Geometry: final body of the model. Coordinates: model frame, mm. A direction names the side the tool comes from. Round coordinates to 2 decimals unless told otherwise and drop trailing zeros. Loops run counter-clockwise (first coordinate to the right, second up) from the corner with the lowest first, then second, coordinate; pieces in that order, holes last. Notation, with made-up numbers: (74.5, 50) - (111.5, 50) arc R20 cw to (111.5, 74) - close; hole circle Ø1 at (68.5, -38). An arc over 180 degrees is marked (long way). Answer as CSV lines item,"result".
Autodesk Inventor part; units mm, degrees
ref_plane "Work Plane1" through (0, 0, 0) normal (0, 0, 1) x (1, 0, 0)
ref_plane "Work Plane2" through (0, 0, 0) normal (0, 0, 1) x (1, 0, 0)
ref_plane "YZ Plane" through (0, 0, 0) normal (1, 0, 0) x (0, 1, 0)
ref_plane "Work Plane1" through (0, 0, 0) normal (0, 0, 1) x (1, 0, 0)
sketch "Sketch1" plane through (0, 0, 0) normal (0, 0, 1) x (1, 0, 0)
  line L0 (-0.2674, 6.35) -> (2.5266, 6.35)
  line L1 (2.5266, 6.35) -> (2.5266, -6.35)
  line L2 (2.9076, -6.35) -> (-0.2674, -6.35)
  line L3 (-0.2674, -6.35) -> (-0.2674, 6.35)
  line L4 (2.5266, -6.35) -> (-0.2674, -6.35)
  line L5 (-0.2674, -6.35) -> (-0.2674, 6.35)
  line L6 (-0.2674, 6.35) -> (2.5266, 6.35)
  line L7 (2.5266, 6.35) -> (2.5266, -6.35)
  point P0 (0, 0)
  dimension "d0" = 2.794
  dimension "d1" = 12.7
extrude "Extrusion1" add sketch "Sketch1" against normal blind 12.7
ref_plane "Work Plane2" through (0, 0, 0) normal (0, 0, 1) x (1, 0, 0)
sketch "Sketch2" plane through (0, 0, 0) normal (0, 0, 1) x (1, 0, 0)
  line L0 (2.9076, -6.35) -> (-0.2674, -6.35)
  line L1 (-0.2674, -6.35) -> (-0.2674, 6.35)
  line L2 (-0.2674, 6.35) -> (2.9076, 6.35)
  line L3 (2.9076, 10.3713) -> (2.9076, 6.35)
  line L4 (2.9076, -6.35) -> (2.9076, -10.3713)
  line L5 (-0.2674, 6.35) -> (-0.2674, -6.35)
  line L6 (-0.2674, -6.35) -> (2.5266, -6.35)
  line L7 (2.5266, -6.35) -> (2.5266, 6.35)
  line L8 (2.5266, 6.35) -> (-0.2674, 6.35)
  line L9 (-0.2674, 6.35) -> (2.9076, 6.35)
  line L10 (2.9076, 6.35) -> (2.9076, -6.35)
  line L11 (2.9076, -6.35) -> (-0.2674, -6.35)
  line L12 (-0.2674, -6.35) -> (-0.2674, 6.35)
  line L13 (6.0826, -12.065) -> (-0.0044, -12.065)
  line L14 (-0.0044, 12.065) -> (6.0826, 12.065)
  line L15 (-2.8074, 9.262) -> (-0.0044, 12.065)
  line L16 (-2.8074, -9.262) -> (-2.8074, 9.262)
  line L17 (-0.0044, -12.065) -> (-2.8074, -9.262)
  line L18 (6.0826, -12.065) -> (6.0826, -10.3713) construction
  line L19 (2.9076, -10.3713) -> (6.0826, -10.3713)
  line L20 (6.0826, 10.3713) -> (2.9076, 10.3713)
  line L21 (6.0826, 10.3713) -> (6.0826, 12.065) construction
  line L22 (2.9076, -10.3713) -> (2.9076, -12.065)
  line L23 (2.9076, 10.3713) -> (2.9076, 12.065)
  point P0 (0, 0)
extrude "Extrusion2" add sketch "Sketch2" along normal blind 3.175
chamfer "Chamfer1" distance 0.635 angle 45 15 edges at (-1.4059, 10.6635, 3.175) (1.4516, 12.065, 3.175) (-2.8074, 0, 3.175) (-1.4059, -10.6635, 3.175) (1.4516, -12.065, 3.175) (1.4516, 12.065, 0) (1.4516, -12.065, 0) (-1.4059, -10.6635, 0) (-2.8074, 0, 0) (-1.4059, 10.6635, 0) (2.9076, 12.065, 1.5875) (2.9076, -12.065, 1.5875) (2.9076, 0, 3.175) (1.1296, 6.35, -12.7) (1.1296, -6.35, -12.7)
properties part number "3114a_Coil Sleeve Lock_V1" material "Acetal Resin, White"
(1) Material intervals for line 1 along X through (y, z) = (4.5, -10.25); line 2 along Y through (x, z) = (-0.1, -9.5); line 3 along Z through (x, y) = (-1.5, 1.75) (3 decimals), sorted ascending.
Findings below:
line 1,"-0.27 to 2.53"
line 2,"-6.35 to 6.35"
line 3,"0 to 3.175"
(2) Section B-B (x = 1.8). Output: boundary loops of the cut face in (y, z) (3 decimals).
Findings below:
outline,"(-12.065, 0.635) - (-11.43, 0) - (-6.35, 0) - (-6.35, -12.065) - (-5.715, -12.7) - (5.715, -12.7) - (6.35, -12.065) - (6.35, 0) - (11.43, 0) - (12.065, 0.635) - (12.065, 2.54) - (11.43, 3.175) - (-11.43, 3.175) - (-12.065, 2.54) - close"
(3) Pin query (flat end, axial travel): P1, Ø2, axis at x = 1, z = -6, coming from the -Y side; P2, Ø5, axis at y = 0.5, z = -11, coming from the +X side; P3, Ø3, axis at x = 0.5, z = -8.5, coming from the +Y side. Return the tip coordinate at first contact, or that it passes through.
Findings below:
P1,"y = -6.35"
P2,"x = 2.53"
P3,"y = 6.35"
(4) Section A-A (y = 1.5). Output: boundary loops of the cut face in (x, z) (3 decimals).
Findings below:
outline,"(-2.807, 0.635) - (-2.172, 0) - (-0.267, 0) - (-0.267, -12.7) - (2.527, -12.7) - (2.527, 0) - (2.908, 0) - (2.908, 2.54) - (2.273, 3.175) - (-2.172, 3.175) - (-2.807, 2.54) - close"
(5) Access query for faces 1 (the face through (1, 6.35, -6)), 2 (the face through (-0.267, 0, -6)), 3 (the face through (2.527, 0, -6)). Directions: +Z, -Z, +X, -X, +Y, -Y. A direction counts if a zero-diameter tool reaches every point of the face in a straight line with its end or side. Return the directions, or none.
Findings below:
face 1,"-Z, +X, -X, +Y"
face 2,"-Z, -X, +Y, -Y"
face 3,"-Z, +X, +Y, -Y"
(6) Section D-D (y = 6.75). Output: boundary loops of the cut face in (x, z) (3 decimals), and give its area (3 significant figures).
Findings below:
outline,"(-2.807, 0.635) - (-2.172, 0) - (2.908, 0) - (2.908, 2.54) - (2.273, 3.175) - (-2.172, 3.175) - (-2.807, 2.54) - close"
area,"17.5 mm2"
(7) Section C-C (z = 1.25). Output: boundary loops of the cut face in (x, y) (3 decimals).
Findings below:
outline,"(-2.807, -9.262) - (-0.004, -12.065) - (2.273, -12.065) - (2.908, -11.43) - (2.908, 11.43) - (2.273, 12.065) - (-0.004, 12.065) - (-2.807, 9.262) - close"
